Autodesk Inventor part; units mm, degrees
ref_plane "YZ Plane" through (0, 0, 0) normal (1, 0, 0) x (0, 1, 0)
ref_plane "XZ Plane" through (0, 0, 0) normal (0, 1, 0) x (-1, 0, 0)
ref_plane "XY Plane" through (0, 0, 0) normal (0, 0, 1) x (1, 0, 0)
sketch "Sketch1" plane through (0, 0, 0) normal (0, 0, 1) x (1, 0, 0)
  line L0 (0, 0) -> (0, 5.2441) construction
  line L1 (0, 0) -> (4.3793, 0) construction
  line L2 (2.9035, 11.25) -> (4.4912, 14)
  line L3 (0.425, 0) -> (0.425, 0.4889) construction
  line L4 (0.425, 0) -> (6.45, 0)
  line L5 (6.45, 0) -> (6.45, 9)
  line L6 (6.45, 9) -> (9, 9)
  line L7 (9, 9) -> (9, 14)
  line L8 (9, 14) -> (4.4912, 14)
  line L9 (0.425, 0) -> (0.425, 2)
  arc A0 (2.9035, 11.25) -> (0.425, 2) centre (18.925, 2) ccw
  dimension "d0" = 0.425
  dimension "d1" = 30
  dimension "d2" = 6.45
  dimension "d3" = 9
  dimension "d4" = 5
  dimension "d6" = 9
  dimension "d14" = 2
  dimension "d15" = 18.5
revolve "Revolution1" add sketch "Sketch1" angle 360 about axis through (0, 0, 0) along (0, 1, 0)
chamfer "Chamfer1" distance 2 angle 45 1 edges at (-9, 9, 0)
chamfer "Chamfer2" distance 2 angle 45 1 edges at (-6.45, 0, 0)
chamfer "Chamfer3" distance 0.5 angle 45 1 edges at (-0.425, 0, 0)
chamfer "Chamfer4" distance 1 angle 45 1 edges at (-9, 14, 0)
properties part number "drop_funnel_v2"
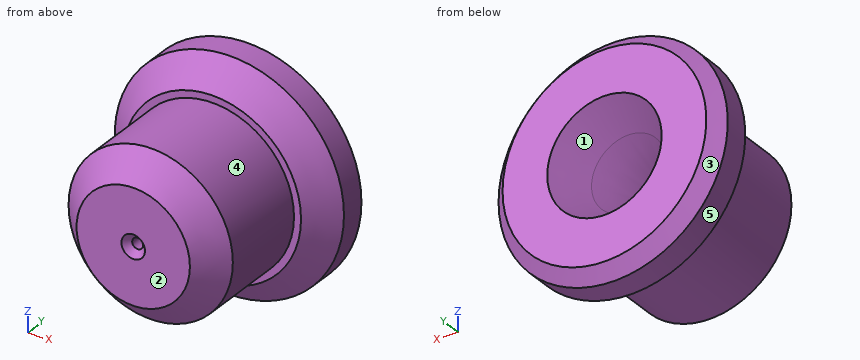
Part model, mm, in its own coordinate system. Face numbers are marked on the shaded views. A direction names the side the tool comes from. Round coordinates to 2 decimals unless told otherwise and drop trailing zeros. Order: outer loops, then holes, each group sorted by start corner. A loop starts at its lowest first (then second) coordinate and runs counter-clockwise, first axis right, second up. Notation, with made-up numbers: (36.5, 26) -> (54.5, 26) arc R26 cw to (54.5, 62) -> close; hole circle Ø3 at (-28.75, 6.5). An arc over 180 degrees is marked (long way). Put each result on its own line as item: value.
Q1. Wall check: line 1 (X direction, y = 1.4, z = 0) (3 decimals); line 2 (Y direction, x = 4.75, z = -2.5); line 3 (Z direction, x = 0, y = 1.25) (3 decimals). Give the ranges that are in metal, low to high. Write a range as [from, to].
From the geometry:
line 1: x = [-5.85, -0.425], [0.425, 5.85]
line 2: y = [0.92, 14]
line 3: z = [-5.7, -0.425], [0.425, 5.7]
Q2. Pull direction Z, two halves, no side cores. Call the marked faces 1, 2 and 3: pulls with the +Z half, pulls with the -Z half, needs draft (parallel to the pull), parting line crosses it, or undercut.
From the geometry:
face 1: undercut
face 2: needs draft
face 3: parting line crosses it
Q3. Band-saw the part on C-C (y = 7.5). Give the cut face in (x, z), and give its area (3 significant figures).
From the geometry:
outline: circle Ø12.9 at (0, 0); hole circle Ø2.52 at (0, 0)
area: 126 mm2
Q4. Tool access for the marked faces 4 and 5: list every direction of +Z, -Z, +X, -X, +Y, -Y with a clear straight run to the whole face (end or side of a thin tool).
From the geometry:
face 4: -Y
face 5: +Y, -Y
Q5. Band-saw the part on D-D (y = 5.75). Give the cut face in (x, z), and give its area (3 significant figures).
From the geometry:
outline: circle Ø12.9 at (0, 0); hole circle Ø1.62 at (0, 0)
area: 129 mm2
Q6. Pin check, flat tips, straight feed: pin 1 Ø1.5 at (y, z) = (12, -2) entering from -X; pin 2 Ø1 at (x, z) = (-2, -1) entering from +Y; pin 3 Ø1 at (y, z) = (12.5, 7) entering from +X. Stop position of each tip, or through.
From the geometry:
pin 1: stops at x = -8.91
pin 2: stops at y = 10.95
pin 3: stops at x = 6.22
